```python
from build123d import *

# Parameters (mm, degrees)
SKETCH2_R            = 2
BOSS_EXTRUDE1_DEPTH  = 17
SKETCH3_R            = 1.5
BOSS_EXTRUDE2_DEPTH  = 7
SKETCH4_W            = 3.988125856
SKETCH4_H            = 4
BOSS_EXTRUDE3_DEPTH  = 2
SKETCH5_W            = 2
SKETCH5_H            = 4
BOSS_EXTRUDE4_DEPTH  = 11
FILLET1_R            = 2
FILLET2_R            = 2
FILLET3_R            = 2
SKETCH6_R            = 1.5
CUT_EXTRUDE1_DEPTH   = 26.709920264
BOSS_EXTRUDE8_START  = -2
BOSS_EXTRUDE8_DEPTH  = 2
SKETCH11_R           = 1.5
BOSS_EXTRUDE9_DEPTH  = 74
SKETCH13_R           = 2
SKETCH13_R_2         = 1.5
BOSS_EXTRUDE10_DEPTH = 3


# Read off the part's stored shape, not the designer's step: Boss-Extrude8
with BuildPart() as part:
    # Sketch2 → Boss-Extrude1 (new body)
    with BuildSketch(Plane(origin=(0, 0, 0), x_dir=(0, 0, -1), z_dir=(1, 0, 0))):
        Circle(SKETCH2_R)
    extrude(amount=BOSS_EXTRUDE1_DEPTH)

    # Sketch3 → Boss-Extrude2 (add)
    with BuildSketch(Plane(origin=(17, 0, 0), x_dir=(0, 0, -1), z_dir=(1, 0, 0))):
        Circle(SKETCH3_R)
    extrude(amount=BOSS_EXTRUDE2_DEPTH)

    # Sketch4 → Boss-Extrude3 (add)
    with BuildSketch(Plane(origin=(24, 0, 0), x_dir=(0, 0, -1), z_dir=(1, 0, 0))):
        with Locations((-0.005937072, 0)):
            Rectangle(SKETCH4_W, SKETCH4_H)
    extrude(amount=-BOSS_EXTRUDE3_DEPTH)

    # Sketch5 → Boss-Extrude4 (add)
    with BuildSketch(Plane.XY.offset(2)):
        with Locations((23, 0)):
            Rectangle(SKETCH5_W, SKETCH5_H)
    extrude(amount=-BOSS_EXTRUDE4_DEPTH)

    # Fillet1
    fillet1_edges = [part.edges().sort_by_distance(p)[0] for p in [
        (23, 2, 2),
    ]]
    fillet(fillet1_edges, radius=FILLET1_R)

    # Fillet2
    fillet2_edges = [part.edges().sort_by_distance(p)[0] for p in [
        (23, -2, 2),
    ]]
    fillet(fillet2_edges, radius=FILLET2_R - 0.0001)  # a hair under: the kernel refuses the full size

    # Fillet3
    fillet3_edges = [part.edges().sort_by_distance(p)[0] for p in [
        (23, -2, -9),
        (23, 2, -9),
    ]]
    fillet(fillet3_edges, radius=FILLET3_R - 0.0001)  # a hair under: the kernel refuses the full size

    # Sketch6 → Cut-Extrude1 (cut, through all)
    with BuildSketch(Plane(origin=(24, 0, 0), x_dir=(0, 0, -1), z_dir=(1, 0, 0))):
        with Locations((7, 0)):
            Circle(SKETCH6_R)
    extrude(amount=-CUT_EXTRUDE1_DEPTH, mode=Mode.SUBTRACT)

    # Boss-Extrude8 outline → Boss-Extrude8 (add)
    with BuildSketch(Plane(origin=(24, 0, 0), x_dir=(0, 0, -1), z_dir=(1, 0, 0)).offset(BOSS_EXTRUDE8_START)):
        with BuildLine():
            Line((7.893788641, 1.789173514), (5.005331724, 3.232113464))
            ThreePointArc((5.005331724, 3.232113464), (3.692949686, 2.855553556), (2.628913929, 2))
            Line((2.628913929, 2), (7, 2))
            ThreePointArc((7, 2), (7.459158453, 1.946579953), (7.893788641, 1.789173514))
        make_face()
        with BuildLine():
            Line((13.26130919, -0.892192368), (7.893788641, 1.789173514))
            ThreePointArc((7.893788641, 1.789173514), (8.701113941, 1.051765829), (9, 0))
            ThreePointArc((9, 0), (8.414213562, -1.414213562), (7, -2))
            Line((7, -2), (6.528240855, -2))
            Line((6.528240855, -2), (11.473731932, -4.470539409))
            ThreePointArc((11.473731932, -4.470539409), (14.156694081, -3.575154517), (13.26130919, -0.892192368))
        make_face()
    extrude(amount=BOSS_EXTRUDE8_DEPTH)

    # Sketch11 → Boss-Extrude9 (add)
    with BuildSketch(Plane(origin=(24, 0, 0), x_dir=(0, 0, -1), z_dir=(1, 0, 0))):
        with Locations((12.367520561, -2.681365888)):
            Circle(SKETCH11_R)
    extrude(amount=BOSS_EXTRUDE9_DEPTH)

    # Sketch13 → Boss-Extrude10 (add)
    # profile 1 of 4: a face of its own
    with BuildSketch(Plane(origin=(98, 0, 0), x_dir=(0, 0, -1), z_dir=(1, 0, 0))):
        with Locations((7, 0)):
            Circle(SKETCH13_R)
        with Locations((7, 0)):
            Circle(SKETCH13_R_2, mode=Mode.SUBTRACT)
    # profile 2 of 4: a face of its own
    with BuildSketch(Plane(origin=(98, 0, 0), x_dir=(0, 0, -1), z_dir=(1, 0, 0))):
        with Locations((12.367520561, -2.681365888)):
            Circle(SKETCH13_R)
        with Locations((12.367520561, -2.681365888)):
            Circle(SKETCH13_R_2, mode=Mode.SUBTRACT)
    # profile 3 of 4: a face of its own
    with BuildSketch(Plane(origin=(98, 0, 0), x_dir=(0, 0, -1), z_dir=(1, 0, 0))):
        with BuildLine():
            ThreePointArc((9, 0), (8.051765834, -1.701113938), (6.106211371, -1.78917352))
            Line((6.106211371, -1.78917352), (11.473731932, -4.470539409))
            ThreePointArc((11.473731932, -4.470539409), (10.578347041, -1.787577259), (13.26130919, -0.892192368))
            Line((13.26130919, -0.892192368), (7.893788629, 1.78917352))
            ThreePointArc((7.893788629, 1.78917352), (8.701113938, 1.051765834), (9, 0))
        make_face()
    # profile 4 of 4: a face of its own
    with BuildSketch(Plane(origin=(98, 0, 0), x_dir=(0, 0, -1), z_dir=(1, 0, 0))):
        with Locations((12.367520561, -2.681365888)):
            Circle(SKETCH13_R_2)
    extrude(amount=BOSS_EXTRUDE10_DEPTH)


solid = part.part
```
The listing builds one solid part. Answer for the finished solid, in the listing's coordinates (mm). A direction names the side the tool comes from. Give positions to 0.01 mm unless a question says otherwise; leave off trailing zeros. Write each loop counter-clockwise with the first axis right and the second up, starting at its lowest first coordinate (ties: lowest second). Pieces come first, ordered by that corner, then holes. Notation, with made-up numbers: (48.5, 18) - (107.5, 18) arc R13 ccw to (107.5, 33) - close; hole circle Ø9 at (-38.75, -17.5). An arc over 180 degrees is marked (long way). Use one line per item in the form item = value. Start each with the question number.
1) Flat-ended cylindrical pins translate along their axes: pin 1 Ø2 at (x, z) = (23.5, -4) entering from -Y; pin 2 Ø1.5 at (x, z) = (24.5, -3.5) entering from +Y; pin 3 Ø0.6 at (x, z) = (23.5, -1) entering from +Y. Find the tip coordinate at first contact, or state that the pin passes through.
2) Consider line 1 along X through (y, z) = (-1, -12.5); line 2 along Y through (x, z) = (33.5, -12.5); line 3 along X through (y, z) = (-0.25, -1). Determine where each line is inside the solid, lowest interval first. Write a range as from..to.
3) Find section A-A on x = 94. Determine the outline of the cut face in (y, z).
4) The mould has two halves that part along Z. Classify faces 1 (the face through (22.99, -3.22, -8.97)), 2 (the face through (98, -1, -10)), 3 (the face through (23.01, 0.07, -5.5)): pulls with the +Z half, pulls with the -Z half, needs draft (parallel to the pull), parting line crosses it, or undercut.
5) A tool of negligible diameter and unlimited length cuts with its end or side. For faces 4 (the face through (8, -2, 0)), 5 (the face through (22.99, -1.4, 1.43)), 6 (the face through (19.46, 0.07, 1.5)), from which of +Z, -Z, +X, -X, +Y, -Y can it reach the whole face along a straight path? Write none if from no direction.
Geometry results:
q1.pin_1 = -2
q1.pin_2 = 3.02
q1.pin_3 = 2
q2.line_1 = 22..24, 98..101
q2.line_2 = -4.18..-1.19
q2.line_3 = 0..24
q3.outline = circle Ø3 at (-2.68, -12.37)
q4.face_1 = pulls with the +Z half
q4.face_2 = needs draft
q4.face_3 = undercut
q5.face_4 = -X
q5.face_5 = +Z, +X, -X, -Y
q5.face_6 = none
